```python
from build123d import *

# Parameters (mm, degrees)
BOSS_EXTRUDE1_DEPTH     = 6.35
FILLET2_R               = 3.175
CUT_EXTRUDE2_DEPTH      = 91.397918676
CUT_EXTRUDE2_DEPTH_BACK = 91.397918676
SKETCH2_R               = 1.5875
SKETCH2_R_2             = 1.4605
CUT_EXTRUDE5_DEPTH      = 91.942464482
CUT_EXTRUDE7_DEPTH      = 25.4
SKETCH6_W               = 10.4785697
SKETCH6_H               = 6.35
SKETCH6_R               = 1.2065
BOSS_EXTRUDE2_DEPTH     = 12.7
FILLET5_R               = 12.7
FILLET6_R               = 5.08
BOSS_EXTRUDE3_DEPTH     = 6.35
SKETCH10_R              = 1.2065
CUT_EXTRUDE9_DEPTH      = 90.841656328


with BuildPart() as part:
    # Sketch1 → Boss-Extrude1 (new body)
    with BuildSketch(Plane(origin=(0, 0, 0), x_dir=(1, 0, 0), z_dir=(0, 1, 0))):
        Polygon((0, 0), (0, 38.989), (-10.16, 38.989), (-71.628, 29.4386), (-81.915, 29.4386), (-81.915, -4.5974), (-71.755, -4.5974), (-10.16, 0), align=None)
    extrude(amount=BOSS_EXTRUDE1_DEPTH)

    # Fillet2
    fillet2_edges = [part.edges().sort_by_distance(p)[0] for p in [
        (0, 0, -19.4945),
        (0, 6.35, -19.4945),
        (-81.915, 0, -12.4206),
        (-81.915, 6.35, -12.4206),
    ]]
    fillet(fillet2_edges, radius=FILLET2_R - 0.0001)  # a hair under: the kernel refuses the full size

    # Sketch2 → Cut-Extrude2 (cut, two sides: drawn at the far end of the back side and taken through both)
    with BuildSketch(Plane(origin=(-0.604981675, 0, 0), x_dir=(-1, 0, 0), z_dir=(0, 0, -1)).offset(-CUT_EXTRUDE2_DEPTH_BACK)):
        with Locations((1.966275702, 3.175)):
            Circle(SKETCH2_R)
        with Locations(Location((77.44064574, 3.175, 0), (0, 0, 180))):
            Circle(SKETCH2_R_2)
    extrude(amount=CUT_EXTRUDE2_DEPTH + CUT_EXTRUDE2_DEPTH_BACK, mode=Mode.SUBTRACT)

    # Sketch3 → Cut-Extrude5 (cut, through all)
    with BuildSketch(Plane(origin=(0, 0, 0), x_dir=(1, 0, 0), z_dir=(0, 1, 0))):
        with BuildLine():
            Line((-81.915, 22.7711), (-71.755, 22.7711))
            Line((-71.755, 22.7711), (-58.487579402, 20.207642468))
            ThreePointArc((-58.487579402, 20.207642468), (-55.580114305, 14.192748547), (-57.777398298, 7.883687982))
            Line((-57.777398298, 7.883687982), (-71.755, 2.0701))
            Line((-71.755, 2.0701), (-81.915, 2.0701))
            Line((-81.915, 2.0701), (-81.915, 22.7711))
        make_face()
        with BuildLine():
            Line((0, 30.5435), (0, 8.4455))
            Line((0, 8.4455), (-7.9756, 8.4455))
            Line((-7.9756, 8.4455), (-17.739567161, 7.096263095))
            Line((-17.739567161, 7.096263095), (-24.764375431, 7.587485542))
            ThreePointArc((-24.764375431, 7.587485542), (-25.820245836, 7.814780317), (-26.769908004, 8.32923828))
            ThreePointArc((-26.769908004, 8.32923828), (-31.345543526, 16.545378703), (-28.210906636, 25.41191441))
            ThreePointArc((-28.210906636, 25.41191441), (-27.55579932, 25.957953915), (-26.795645997, 26.34459543))
            Line((-26.795645997, 26.34459543), (-15.585156538, 30.5435))
            Line((-15.585156538, 30.5435), (-7.9756, 30.5435))
            Line((-7.9756, 30.5435), (0, 30.5435))
        make_face()
    extrude(amount=CUT_EXTRUDE5_DEPTH, mode=Mode.SUBTRACT)

    # Sketch5 → Cut-Extrude7 (cut)
    with BuildSketch(Plane(origin=(0, 6.35, 0), x_dir=(1, 0, 0), z_dir=(0, 1, 0))):
        Polygon((-10.16, 38.989), (-53.78735915, 28.179846815), (-71.628, 29.4386), align=None)
        Polygon((-10.16, 0), (-47.394119509, 2.627067431), (-71.755, -4.5974), align=None)
    extrude(amount=-CUT_EXTRUDE7_DEPTH, mode=Mode.SUBTRACT)

    # Sketch6 → Boss-Extrude2 (add)
    with BuildSketch(Plane.XY.offset(-31.75)):
        with Locations((-43.810886798, 3.175)):
            Rectangle(SKETCH6_W, SKETCH6_H)
        with Locations((-45.72, 3.108706623)):
            Circle(SKETCH6_R, mode=Mode.SUBTRACT)
        with Locations((-42.164, 3.108706623)):
            Circle(SKETCH6_R, mode=Mode.SUBTRACT)
    extrude(amount=BOSS_EXTRUDE2_DEPTH)

    # Fillet5
    fillet5_edges = [part.edges().sort_by_distance(p)[0] for p in [
        (-53.78735915, 3.175, -28.179846815),
        (-47.394119509, 3.175, -2.627067431),
    ]]
    fillet(fillet5_edges, radius=FILLET5_R)

    # Fillet6
    fillet6_edges = [part.edges().sort_by_distance(p)[0] for p in [
        (-57.777398298, 3.175, -7.883687982),
        (-58.487579402, 3.175, -20.207642468),
    ]]
    fillet(fillet6_edges, radius=FILLET6_R)

    # Sketch9 → Boss-Extrude3 (add)
    with BuildSketch(Plane(origin=(0, 6.35, 0), x_dir=(1, 0, 0), z_dir=(0, 1, 0))):
        Polygon((-49.050171648, 31.75), (-71.628, 29.4386), (-71.628, 26.697361781), (-49.050171648, 26.697361781), align=None)
    extrude(amount=-BOSS_EXTRUDE3_DEPTH)

    # Sketch10 → Cut-Extrude9 (cut, through all)
    with BuildSketch(Plane(origin=(0, 0, -31.75), x_dir=(-1, 0, 0), z_dir=(0, 0, -1))):
        with Locations((42.164, 3.108706623)):
            Circle(SKETCH10_R)
        with Locations(Location((45.72, 3.108706623, 0), (0, 0, 121.083308631))):
            Circle(SKETCH10_R)
    extrude(amount=-CUT_EXTRUDE9_DEPTH, mode=Mode.SUBTRACT)


solid = part.part
```
Here's how the part is built. I have some questions about the finished solid (model axes, mm). A direction names the side the tool comes from. Give positions to 0.01 mm unless a question says otherwise; leave off trailing zeros. Loops run counter-clockwise (first coordinate to the right, second up) from the corner with the lowest first, then second, coordinate; pieces in that order, holes last. Notation, with made-up numbers: M 7,59.5 L 32,59.5 A9 ccw 32,68.5 Z; hole C 53,-8.75 d11. An arc over 180 degrees is marked long. Put each result on its own line as item: value. Start each with the question number.
(1) I want a section at C-C on x = -74. Please give me the cut outline in (y, z).
(2) Will these pins go through, and if not, where does the flat tip stop? pin 1 Ø3 at (x, y) = (-74.5, 3.5) entering from -Z; pin 2 Ø3 at (x, y) = (-45.72, 3.11) entering from -Z; pin 3 Ø2 at (y, z) = (5.5, -13.5) entering from +X.
(3) For faces 1 (the flat face through (-65.34, 3.13, -4.74)), 2 (the cylindrical face through (-25.81, 3.13, -7.81)), 3 (the flat face through (-44, 3, -31.75)), 4 (the flat face through (-8, 3, -30.544)), which set-ups out of +Z, -Z, +X, -X, +Y, -Y let a thin tool reach every point of the face, with its end or its side?
(4) If we mould it in two halves opening along Y, with no side actions, what happens to faces 5 (the cylindrical face through (-3.425, 4.514, -4.164)), 6 (the flat face through (-6, 3, -38.989)), 7 (the cylindrical face through (-0.91, 0.95, -4.28))? For each: +Y half, -Y half, draft (parallel to the pull), parting line (faces both ways), or undercut.
(5) I want a section at A-A on x = -6.5. Please give me the cut outline in (y, z).
(6) I want a section at B-B on z = -4. State how many separate pieces and enclosed holes the cut face has, then the cut area to 3 significant figures.
(7) I need wall thicknesses on line 1 along Z through (x, y) = (-75, 2.5); line 2 along X through (y, z) = (2.5, -10); line 3 along Z through (x, y) = (-41, 5.25). Which ranges of each line are inside material? Lowest first, please. Write a range as [from, to].
Answer block:
1. outline: M 0,-29.44 L 6.35,-29.44 L 6.35,-22.77 L 0,-22.77 Z; M 0,-2.07 L 6.35,-2.07 L 6.35,4.6 L 0,4.6 Z
2. pin 1: z = -29.44
2. pin 2: z = -31.75
2. pin 3: x = -30.23
3. face 1: -X, +Y, -Y
3. face 2: +Y, -Y
3. face 3: -Z, -X, +Y, -Y
3. face 4: +X, +Y, -Y
4. face 5: undercut
4. face 6: draft
4. face 7: -Y half
5. outline: M 0,-38.99 L 6.35,-38.99 L 6.35,-30.54 L 0,-30.54 Z; M 0,-8.45 L 6.35,-8.45 L 6.35,0 L 0,0 Z
6. separate pieces: 1
6. enclosed holes: 3
6. area: 405 mm^2
7. line 1: [-29.44, -22.77], [-2.07, 4.6]
7. line 2: [-56.38, -46.76], [-44.68, -43.21], [-41.12, -28.58]
7. line 3: [-31.75, -2.18]
